Autodesk Inventor part; units mm, degrees
ref_plane "YZ Plane" through (0, 0, 0) normal (1, 0, 0) x (0, 1, 0)
ref_plane "XZ Plane" through (0, 0, 0) normal (0, 1, 0) x (-1, 0, 0)
ref_plane "XY Plane" through (0, 0, 0) normal (0, 0, 1) x (1, 0, 0)
sketch "Szkic2" plane through (0, 0, 0) normal (1, 0, 0) x (0, 1, 0)
  line L0 (0, -2.9) -> (0, 2.9)
  line L1 (-1.5, -1.5) -> (-1.5, 1.5)
  line L2 (-1.5, -1.5) -> (0, -2.9)
  line L3 (-1.5, 1.5) -> (0, 2.9)
  line L4 (0, 0) -> (-18, 0)
  line L5 (-18, 0) -> (-18, -1.5)
  line L6 (-18, -1.5) -> (-1.5, -1.5)
  dimension "d0" = 5.8
  dimension "d2" = 3
  dimension "d3" = 1.5
  dimension "d4" = 18
  dimension "d5" = 1.5
revolve "Obrót1" add sketch "Szkic2" angle 360 about axis through (0, 0, 0) along (0, -1, 0) contours L2 L1 L4 L0 | L6 L5 L4 L1
sketch "Szkic3" plane through (0, 0, 0) normal (0, 1, 0) x (1, 0, 0)
  line L0 (-1.1673, -0.633) -> (-1.1318, 0.6945)
  line L1 (-1.1318, 0.6945) -> (0.0355, 1.3274)
  line L2 (0.0355, 1.3274) -> (1.1673, 0.633)
  line L3 (1.1673, 0.633) -> (1.1318, -0.6945)
  line L4 (1.1318, -0.6945) -> (-0.0355, -1.3274)
  line L5 (-0.0355, -1.3274) -> (-1.1673, -0.633)
  point P0 (0, 0)
  point P1 (0, 0)
  dimension "d7" = 2.3
extrude "Wyciągnięcie proste1" cut sketch "Szkic3" against normal blind 2
fillet "Zaokrąglenie1" radius 0.5 6 edges at (-1.1496, -2, -0.0308) (-0.6014, -2, 0.9802) (-0.5482, -2, -1.011) (0.6014, -2, -0.9802) (0.5482, -2, 1.011) (1.1496, -2, 0.0308)
fillet "Zaokrąglenie2" radius 0.5 1 edges at (0, -1.5, 1.5)
fillet "Zaokrąglenie3" radius 0.1 1 edges at (0, 0, 2.9)
thread "Gwint1"
chamfer "Faza1" distance 0.5 angle 45 1 edges at (0, -18, 1.5)
properties part number "Screw M3 18mm flat head"
Geometry: final body of the model. Coordinates: model frame, mm. A direction names the side the tool comes from. Coordinates: 2 decimals unless noted, no trailing zeros. Loops run counter-clockwise (first coordinate to the right, second up) from the corner with the lowest first, then second, coordinate; pieces in that order, holes last. Notation, with made-up numbers: (-12.75, 28) - (11.25, 28) arc R32 ccw to (11.25, 54) - close; hole circle Ø7 at (73, 60.25). An arc over 180 degrees is marked (long way). One line per question, with ' | ' between items. Start each with the question number.
(1) Draft query along Z for faces 1 (the flat face through (-1, 0, -1)), 2 (the cylindrical face through (-0.47, -1.86, -0.88)), 3 (the cylindrical face through (-0.07, -9.49, 1.5)). Return one class per face: +Z half, -Z half, draft (parallel to the pull), parting line (faces both ways), or undercut.
(2) Ray query, L1, parallel to Z at x = 1.3, y = -2; L2, parallel to Z at x = 0.1, y = -0.75; L3, parallel to Z at x = 1, y = -1.75. Return the intervals inside material, ascending. Write a range as from..to.
(3) Cut plane A-A on y = -8.75. Output: boundary loops of the cut face in (x, z).
(4) First-contact query: pin 1 (1.5 mm diameter, centred on y = -6.5, z = 1, fed in from -X); pin 2 (3 mm diameter, centred on y = -4.5, z = 1, fed in from +X); pin 3 (0.7 mm diameter, centred on x = 0, z = 0.5, fed in from +Y). Flat tips, straight axial feed; report the tip coordinate or a pass-through.
(5) Reachability of faces 4 (the flat face through (0, -18, 0)), 5 (the flat face through (-0.593, -0.74, 0.985)) from +Z, -Z, +X, -X, +Y, -Y: full face, straight path, thin tool, end or side. Return the list, or none.
Here are the results:
1) face 1: draft | face 2: undercut | face 3: parting line
2) L1: -0.75..0.75 | L2: -2.2..-1.29, 1.25..2.2 | L3: -1.12..-0.66, 0.69..1.12
3) outline: circle Ø3 at (0, 0)
4) pin 1: x = -1.48 | pin 2: x = 1.5 | pin 3: y = -1.98
5) face 4: +Z, -Z, +X, -X, -Y | face 5: +Y
